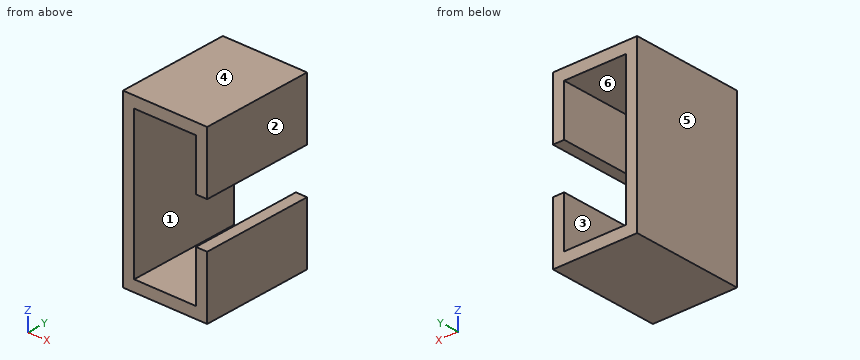
from build123d import *

# Parameters (mm, degrees)
F1_DEPTH = 25.4
F2_T     = -2.54
F3_DEPTH = 25.4
F4_W     = 2.54
F4_H     = 10.16
F5_DEPTH = 25.4


with BuildPart() as f1:
    # F0 (on Front) → F1 (new body)
    with BuildSketch(Plane.XZ):
        Polygon((0, -8.89), (0, 8.89), (0, 19.05), (-19.05, 19.05), (-19.05, 0), (-19.05, -19.05), (0, -19.05), align=None)
    extrude(amount=F1_DEPTH)

    # F2
    f2_openings = [f1.faces().sort_by_distance(p)[0] for p in [
        (-9.525, -25.4, 0),
    ]]
    offset(amount=F2_T, openings=f2_openings)

    # F3 (cut): a face of the model
    f3_faces = [f1.faces().sort_by_distance(p)[0] for p in [
        (-9.525, -2.54, 0),
    ]]
    extrude(f3_faces, amount=-F3_DEPTH, mode=Mode.SUBTRACT)

    # F4 (on face) → F5 (cut)
    with BuildSketch(Plane.XZ.offset(25.4)):
        with Locations((-1.27, 0)):
            Rectangle(F4_W, F4_H)
    extrude(amount=-F5_DEPTH, mode=Mode.SUBTRACT)


solid = f1.part
Part model, mm, in its own coordinate system. Face numbers are marked on the shaded views. A direction names the side the tool comes from. Coordinates: 2 decimals unless noted, no trailing zeros. Write each loop counter-clockwise with the first axis right and the second up, starting at its lowest first coordinate (ties: lowest second). Pieces come first, ordered by that corner, then holes. Notation, with made-up numbers: M 38.5,43.5 L 43.5,43.5 A27 cw 43.5,72.5 Z; hole C 57,3.5 d8. An arc over 180 degrees is marked long. Return JSON: item names as keys, results as strings.
1. Probe L1, parallel to Z at x = -14.25, y = -18; L2, parallel to X at y = -15.75, z = -9.5; L3, parallel to X at y = -9.25, z = 4.5. List the from-to ranges inside material, lowest first.
Determined:
{"L1": "-19.05 to -16.51, 16.51 to 19.05", "L2": "-19.05 to -16.51, -2.54 to 0", "L3": "-19.05 to -16.51"}
2. Flat gauge pins, fed straight in: pin 1 Ø8 at (x, z) = (-14, 10) entering from +Y; pin 2 Ø1 at (x, z) = (-10, -15) entering from -Y. Where does each tip first touch, or does it go through?
Determined:
{"pin 1": "y = 0", "pin 2": "through"}
3. 3-axis set-ups, long thin cutter, end or side, ignore diameter. For the marked faces 5 and 6: which of +Z, -Z, +X, -X, +Y, -Y reach the whole face in a straight line?
Determined:
{"face 5": "+Z, -Z, -X, +Y, -Y", "face 6": "+Y, -Y"}
4. Saw through at C-C, the plane y = -17.25. Write the cut outline in (x, z).
Determined:
{"outline": "M -19.05,-19.05 L 0,-19.05 L 0,-5.08 L -2.54,-5.08 L -2.54,-16.51 L -16.51,-16.51 L -16.51,16.51 L -2.54,16.51 L -2.54,5.08 L 0,5.08 L 0,19.05 L -19.05,19.05 Z"}
5. Saw through at B-B, the plane z = -7.5. Write the cut outline in (x, y), then the cut area to 3 significant figures.
Determined:
{"outline": "M -19.05,-25.4 L -16.51,-25.4 L -16.51,0 L -19.05,0 Z; M -2.54,-25.4 L 0,-25.4 L 0,0 L -2.54,0 Z", "area": "129 mm²"}
6. Pull direction Z, two halves, no side cores. Call the marked faces 1, 2, 3 and 4: pulls with the +Z half, pulls with the -Z half, needs draft (parallel to the pull), parting line crosses it, or undercut.
Determined:
{"face 1": "undercut", "face 2": "needs draft", "face 3": "undercut", "face 4": "pulls with the +Z half"}
7. Saw through at A-A, the plane x = -9.25. Write the cut outline in (y, z), then the cut area to 3 significant figures.
Determined:
{"outline": "M -25.4,-19.05 L 0,-19.05 L 0,-16.51 L -25.4,-16.51 Z; M -25.4,16.51 L 0,16.51 L 0,19.05 L -25.4,19.05 Z", "area": "129 mm²"}
